from build123d import *

# Parameters (mm, degrees)
EXTRUDE_1_DEPTH     = 30
SKETCH_2_R          = 3
CUT_EXTRUDE_1_DEPTH = 5


with BuildPart() as part:
    # 草图1 → 凸台-拉伸1 (new body)
    with BuildSketch(Plane(origin=(0, 0, 0), x_dir=(0, 0, -1), z_dir=(1, 0, 0))):
        with BuildLine():
            Line((-14, 10.127016654), (-14, -10.127016654))
            ThreePointArc((-14, -10.127016654), (-13.790569415, -10.739389089), (-13.25, -11.09526249))
            ThreePointArc((-13.25, -11.09526249), (-11.878679656, -11.878679656), (-11.09526249, -13.25))
            ThreePointArc((-11.09526249, -13.25), (-10.739389089, -13.790569415), (-10.127016654, -14))
            Line((-10.127016654, -14), (10.127016654, -14))
            ThreePointArc((10.127016654, -14), (10.739389089, -13.790569415), (11.09526249, -13.25))
            ThreePointArc((11.09526249, -13.25), (11.878679656, -11.878679656), (13.25, -11.09526249))
            ThreePointArc((13.25, -11.09526249), (13.790569415, -10.739389089), (14, -10.127016654))
            Line((14, -10.127016654), (14, 10.127016654))
            ThreePointArc((14, 10.127016654), (13.790569415, 10.739389089), (13.25, 11.09526249))
            ThreePointArc((13.25, 11.09526249), (11.878679656, 11.878679656), (11.09526249, 13.25))
            ThreePointArc((11.09526249, 13.25), (10.739389089, 13.790569415), (10.127016654, 14))
            Line((10.127016654, 14), (-10.127016654, 14))
            ThreePointArc((-10.127016654, 14), (-10.739389089, 13.790569415), (-11.09526249, 13.25))
            ThreePointArc((-11.09526249, 13.25), (-11.878679656, 11.878679656), (-13.25, 11.09526249))
            ThreePointArc((-13.25, 11.09526249), (-13.790569415, 10.739389089), (-14, 10.127016654))
        make_face()
    extrude(amount=-EXTRUDE_1_DEPTH)

    # 草图2 → 切除-拉伸1 (cut)
    with BuildSketch(Plane(origin=(0, 0, 0), x_dir=(0, 0, -1), z_dir=(1, 0, 0))):
        Circle(SKETCH_2_R)
    extrude(amount=-CUT_EXTRUDE_1_DEPTH, mode=Mode.SUBTRACT)


solid = part.part
Here's how the part is built. I have some questions about the finished solid (model axes, mm). A direction names the side the tool comes from. Coordinates: 2 decimals unless noted, no trailing zeros. Write each loop counter-clockwise with the first axis right and the second up, starting at its lowest first coordinate (ties: lowest second). Pieces come first, ordered by that corner, then holes. Notation, with made-up numbers: (35, -29.75) - (68, -29.75) arc R29 cw to (68, 0.25) - close; hole circle Ø5 at (1, 67.5). An arc over 180 degrees is marked (long way). Use one line per item in the form item = value.
1) Suppose I cut it at A-A, the plane y = 0. Write out the boundary of the cut face in (x, z).
Solved:
outline = (-30, -14) - (0, -14) - (0, -3) - (-5, -3) - (-5, 3) - (0, 3) - (0, 14) - (-30, 14) - close
2) Suppose I cut it at C-C, the plane x = -7. Write out the boundary of the cut face in (y, z).
Solved:
outline = (-14, -10.13) arc R1 ccw to (-13.25, -11.1) arc R3 cw to (-11.1, -13.25) arc R1 ccw to (-10.13, -14) - (10.13, -14) arc R1 ccw to (11.1, -13.25) arc R3 cw to (13.25, -11.1) arc R1 ccw to (14, -10.13) - (14, 10.13) arc R1 ccw to (13.25, 11.1) arc R3 cw to (11.1, 13.25) arc R1 ccw to (10.13, 14) - (-10.13, 14) arc R1 ccw to (-11.1, 13.25) arc R3 cw to (-13.25, 11.1) arc R1 ccw to (-14, 10.13) - close
3) I'm going to push a flat-ended pin straight in: P1, Ø1.8, axis at y = -0.5, z = 1.5, coming from the +X side. Where does the tip first touch, or does it pass through?
Solved:
P1 = -5
4) I need wall thicknesses on line 1 (Y direction, x = -1.15, z = 0); line 2 (Y direction, x = -3.5, z = 0.75); line 3 (X direction, y = 1.25, z = -2.5). Which ranges of each line are inside material? Lowest first, please.
Solved:
line_1 = -14 to -3, 3 to 14
line_2 = -14 to -2.9, 2.9 to 14
line_3 = -30 to -5
5) Suppose I cut it at D-D, the plane y = -11.5. Write out the boundary of the cut face in (x, z).
Solved:
outline = (-30, -12.34) - (0, -12.34) - (0, 12.34) - (-30, 12.34) - close
6) Thinking about a two-plate mould opening in Z: for faces 1 (the cylindrical face through (-14.79, -13.8, -10.73)), 2 (the cylindrical face through (-2, 0, 3)), 3 (the flat face through (-15, 14, 0)), which applies, released by +Z, released by -Z, zero draft, split by the parting line, or undercut?
Solved:
face_1 = released by -Z
face_2 = undercut
face_3 = zero draft
7) On a 3-axis mill with a long thin cutter (end or side, diameter ignored), from which of +Z, -Z, +X, -X, +Y, -Y can I reach the whole of each face in a straight line? I mean faces 4 (the flat face through (-5, 0, 0)), 5 (the cylindrical face through (-14.79, 13.8, 10.73)). Say none if no direction works.
Solved:
face_4 = +X
face_5 = +Z, +X, -X, +Y
